The listing builds one solid part. Answer for the finished solid, in the listing's coordinates (mm). Face numbers are marked on the shaded views. A direction names the side the tool comes from. Round coordinates to 2 decimals unless told otherwise and drop trailing zeros. Write each loop counter-clockwise with the first axis right and the second up, starting at its lowest first coordinate (ties: lowest second). Pieces come first, ordered by that corner, then holes. Notation, with made-up numbers: M -29,15 L 0,15 A26 ccw 0,36 Z; hole C 53,85.25 d6. An arc over 180 degrees is marked long. One line per item, written item: value. Start each with the question number.
(1) Section D-D (y = 22.5) is taken. State how many separate pieces and enclosed holes the cut face has, plus the area to 3 significant figures.
(2) Section C-C (z = 0) is taken. Determine the outline of the cut face in (x, y), plus the area to 3 significant figures.
(3) For the marked faces 4, 5 and 6, determine the directions among +Z, -Z, +X, -X, +Y, -Y from which every point of the face is accessible in a straight line to the end or side of a thin tool.
(4) Consider probe 1 along Z at (x, y) = (-6, 9); probe 2 along Z at (x, y) = (-9.5, 1); probe 3 along Y at (x, z) = (0, -28.4). Determine where each line is inside the solid, lowest interval first.
(5) For a pull along Z with two mould halves and no side action, classify the marked faces 1, 2 and 3 as released by +Z, released by -Z, zero draft, split by the parting line, or undercut.
(6) Given P1, Ø5.5, axis at x = -11, z = -20, coming from the -Y side; P2, Ø5.5, axis at y = -1.5, z = -19.5, coming from the +X side; P3, Ø3, axis at x = 11, z = -20, coming from the +Y side, each flat-ended and moving along its own axis, determine where each tip first touches the part or whether it passes through.
(7) Section A-A (z = -20) is taken. Determine the outline of the cut face in (x, y), plus the area to 3 significant figures.
(8) Section B-B (x = -11) is taken. Determine the outline of the cut face in (y, z), plus the area to 3 significant figures.
```python
from build123d import *

# Parameters (mm, degrees)
SKETCH1_W           = 30
SKETCH1_H           = 60
BOSS_EXTRUDE1_DEPTH = 5
SKETCH3_R           = 3.5
BOSS_EXTRUDE2_DEPTH = 6.9
SKETCH4_R           = 7.7
CUT_EXTRUDE1_DEPTH  = 1.5
SKETCH6_R           = 6.7
CUT_EXTRUDE2_DEPTH  = 3.5
SKETCH9_R           = 4.75
CUT_EXTRUDE4_DEPTH  = 0.6
FILLET1_R           = 15
SKETCH15_R          = 1.65
CUT_EXTRUDE5_DEPTH  = 10
SKETCH16_W          = 15
SKETCH16_H          = 6.25
BOSS_EXTRUDE3_DEPTH = 5
FILLET2_R           = 1.5
FILLET3_R           = 1


with BuildPart() as part:
    # Sketch1 → Boss-Extrude1 (new body)
    with BuildSketch(Plane(origin=(0, 0, 0), x_dir=(1, 0, 0), z_dir=(0, 1, 0))):
        Rectangle(SKETCH1_W, SKETCH1_H)
    extrude(amount=BOSS_EXTRUDE1_DEPTH)

    # Sketch3 → Boss-Extrude2 (add)
    with BuildSketch(Plane.XY.offset(30)):
        Polygon((-15, 5), (15, 5), (15, 25), (15, 40), (-15, 40), (-15, 25), align=None)
        with Locations((0, 25)):
            Circle(SKETCH3_R, mode=Mode.SUBTRACT)
    boss_extrude2 = extrude(amount=-BOSS_EXTRUDE2_DEPTH)

    # Sketch4 → Cut-Extrude1 (cut)
    with BuildSketch(Plane(origin=(0, 0, 23.1), x_dir=(-1, 0, 0), z_dir=(0, 0, -1))):
        with Locations((0, 25)):
            Circle(SKETCH4_R)
    cut_extrude1 = extrude(amount=-CUT_EXTRUDE1_DEPTH, mode=Mode.SUBTRACT)

    # Sketch6 → Cut-Extrude2 (cut)
    with BuildSketch(Plane(origin=(0, 0, 24.6), x_dir=(-1, 0, 0), z_dir=(0, 0, -1))):
        with Locations((0, 25)):
            Circle(SKETCH6_R)
    cut_extrude2 = extrude(amount=-CUT_EXTRUDE2_DEPTH, mode=Mode.SUBTRACT)

    # Sketch9 → Cut-Extrude4 (cut)
    with BuildSketch(Plane(origin=(0, 0, 28.1), x_dir=(-1, 0, 0), z_dir=(0, 0, -1))):
        with Locations((0, 25)):
            Circle(SKETCH9_R)
    cut_extrude4 = extrude(amount=-CUT_EXTRUDE4_DEPTH, mode=Mode.SUBTRACT)

    # Mirror2: Boss-Extrude2, Cut-Extrude1, Cut-Extrude2, Cut-Extrude4 across plane
    add(boss_extrude2.mirror(Plane.XY))
    add(cut_extrude1.mirror(Plane.XY), mode=Mode.SUBTRACT)
    add(cut_extrude2.mirror(Plane.XY), mode=Mode.SUBTRACT)
    add(cut_extrude4.mirror(Plane.XY), mode=Mode.SUBTRACT)

    # Fillet1
    fillet1_edges = [part.edges().sort_by_distance(p)[0] for p in [
        (-15, 40, -26.55),
        (15, 40, -26.55),
        (-15, 40, 26.55),
        (15, 40, 26.55),
    ]]
    fillet(fillet1_edges, radius=FILLET1_R - 0.0001)  # a hair under: the kernel refuses the full size

    # Sketch15 → Cut-Extrude5 (cut)
    with BuildSketch(Plane(origin=(0, 5, 0), x_dir=(1, 0, 0), z_dir=(0, 1, 0))):
        with Locations(Location((-11, -20, 0), (0, 0, 270))):
            Circle(SKETCH15_R)
        with Locations(Location((11, -20, 0), (0, 0, 270))):
            Circle(SKETCH15_R)
        with Locations(Location((-11, 20, 0), (0, 0, 270))):
            Circle(SKETCH15_R)
        with Locations(Location((11, 20, 0), (0, 0, 270))):
            Circle(SKETCH15_R)
    extrude(amount=-CUT_EXTRUDE5_DEPTH, mode=Mode.SUBTRACT)

    # Sketch16 → Boss-Extrude3 (add)
    with BuildSketch(Plane.XZ):
        with Locations((0, 20)):
            Rectangle(SKETCH16_W, SKETCH16_H)
        with Locations((0, -20)):
            Rectangle(SKETCH16_W, SKETCH16_H)
    extrude(amount=BOSS_EXTRUDE3_DEPTH)

    # Fillet2
    fillet2_edges = [part.edges().sort_by_distance(p)[0] for p in [
        (0, 0, -30),
        (0, 0, 30),
    ]]
    fillet(fillet2_edges, radius=FILLET2_R)

    # Fillet3
    fillet3_edges = [part.edges().sort_by_distance(p)[0] for p in [
        (0, -5, 23.125),
        (0, -5, 16.875),
        (0, -5, -16.875),
        (0, -5, -23.125),
    ]]
    fillet(fillet3_edges, radius=FILLET3_R)


solid = part.part
```
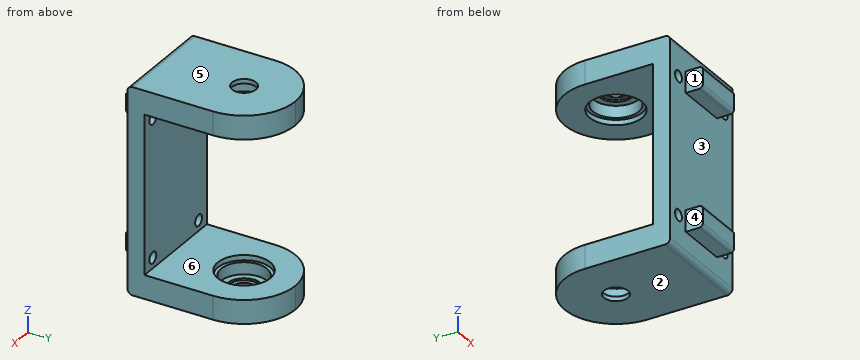
Recorded:
1. separate pieces: 4
1. enclosed holes: 0
1. area: 261 mm2
2. outline: M -15,0 L 15,0 L 15,5 L -15,5 Z
2. area: 150 mm2
3. face 4: +Z, -Z, -X, -Y
3. face 5: +Z, +X, -X, +Y, -Y
3. face 6: +X, -X, +Y
4. probe 1: z = -30 to -23.1, 23.1 to 30
4. probe 2: z = -29.91 to -20.69, -19.31 to 19.31, 20.69 to 29.91
4. probe 3: y = 0 to 20.25, 29.75 to 40
5. face 1: zero draft
5. face 2: released by -Z
5. face 3: undercut
6. P1: stops at y = 0
6. P2: stops at x = 15
6. P3: passes through
7. outline: M -15,0 L -12.65,0 L -12.65,5 L -15,5 Z; M -9.35,0 L -7.5,0 L -7.5,-5 L 7.5,-5 L 7.5,0 L 9.35,0 L 9.35,5 L -9.35,5 Z; M 12.65,0 L 15,0 L 15,5 L 12.65,5 Z
7. area: 192 mm2
8. outline: M 0,-28.5 A1.5 ccw 1.5,-30 L 35.2,-30 L 35.2,-23.1 L 5,-23.1 L 5,-21.65 L 0,-21.65 Z; M 0,-18.35 L 5,-18.35 L 5,18.35 L 0,18.35 Z; M 0,21.65 L 5,21.65 L 5,23.1 L 35.2,23.1 L 35.2,30 L 1.5,30 A1.5 ccw 0,28.5 Z
8. area: 683 mm2
